Could you check a few things on this model? Use its own coordinates, in mm. Coordinates: 2 decimals unless noted, no trailing zeros. Loops run counter-clockwise (first coordinate to the right, second up) from the corner with the lowest first, then second, coordinate; pieces in that order, holes last. Notation, with made-up numbers: (21, 63) - (74, 63) arc R30 cw to (74, 97) - close; hole circle Ø1 at (75.25, 54.25). An arc over 180 degrees is marked (long way). One line per item, written item: value. Start each with the question number.
(1) If I drill on line 1 along Y through (x, z) = (1324, 0.2); line 2 along X through (y, z) = (-100.25, 1.1); line 3 along X through (y, z) = (-99.25, 0.5), over which ranges is the centre line in solid material (lowest first)? Write a range as from..to.
(2) I'm going to push flat-ended pins straight in: P1, Ø0.9, axis at x = 1324, z = 2, coming from the +Y side; P2, Ø1.5, axis at x = 1284.5, z = 2, coming from the -Y side. Where does each tip first touch, or does it pass through?
(3) If we section it at C-C on x = 1315: Write out the boundary of the cut face in (y, z), then the cut area to 3 significant figures.
(4) If we section it at A-A on z = 0.55: Write out the boundary of the cut face in (x, y).
(5) If we section it at B-B on x = 1269: Write out the boundary of the cut face in (y, z), then the cut area to 3 significant figures.
```python
from build123d import *

# Parameters (mm, degrees)
SKETCH1_R          = 2.314653827
BASE_EXTRUDE_DEPTH = 3


with BuildPart() as part:
    # Sketch1 → Base-Extrude (new body)
    with BuildSketch(Plane.XY):
        with BuildLine():
            Line((1237.912051302, -106.965442143), (1245.987496986, -95.560571197))
            ThreePointArc((1245.987496986, -95.560571197), (1253.509408231, -96.263863256), (1254.634364731, -103.73435463))
            Line((1254.634364731, -103.73435463), (1304.653724872, -103.73435463))
            Line((1304.653724872, -103.73435463), (1317.227321876, -96.706912395))
            Line((1317.227321876, -96.706912395), (1326.560817804, -96.706912395))
            Line((1326.560817804, -96.706912395), (1329.452389013, -100.73435463))
            Line((1329.452389013, -100.73435463), (1321.620543519, -100.73435463))
            Line((1321.620543519, -100.73435463), (1321.620543519, -103.73435463))
            Line((1321.620543519, -103.73435463), (1356.049186006, -103.73435463))
            ThreePointArc((1356.049186006, -103.73435463), (1359.51702166, -102.336314635), (1361.045588138, -98.92400098))
            Line((1361.045588138, -98.92400098), (1361.062528583, -98.477689842))
            Line((1361.062528583, -98.477689842), (1361.062528583, -98.158287995))
            ThreePointArc((1361.062528583, -98.158287995), (1361.210092551, -97.803620765), (1361.565683957, -97.658297951))
            Line((1361.565683957, -97.658297951), (1365.63036841, -97.683949663))
            Line((1365.63036841, -97.683949663), (1365.576237812, -106.261303213))
            Line((1365.576237812, -106.261303213), (1368.576237812, -106.280235835))
            Line((1368.576237812, -106.280235835), (1368.620142395, -99.323262365))
            Line((1368.620142395, -99.323262365), (1372.856385089, -99.349996759))
            ThreePointArc((1372.856385089, -99.349996759), (1375.348322676, -105.366702643), (1372.855935111, -111.383222141))
            Line((1372.855935111, -111.383222141), (1255.179553467, -111.383222141))
            ThreePointArc((1255.179553467, -111.383222141), (1248.674645996, -113.340903741), (1241.936111152, -114.200256171))
            Line((1241.936111152, -114.200256171), (1245.086093213, -109.745869716))
            Line((1245.086093213, -109.745869716), (1242.636669623, -108.013725357))
            Line((1242.636669623, -108.013725357), (1239.591696444, -112.41591336))
            Line((1239.591696444, -112.41591336), (1238.460322727, -110.884264434))
            Line((1238.460322727, -110.884264434), (1237.923801474, -109.055713836))
            Line((1237.923801474, -109.055713836), (1237.912051302, -106.965442143))
        make_face()
        with Locations((1249.299132798, -100.717822078)):
            Circle(SKETCH1_R, mode=Mode.SUBTRACT)
    extrude(amount=BASE_EXTRUDE_DEPTH)


solid = part.part
```
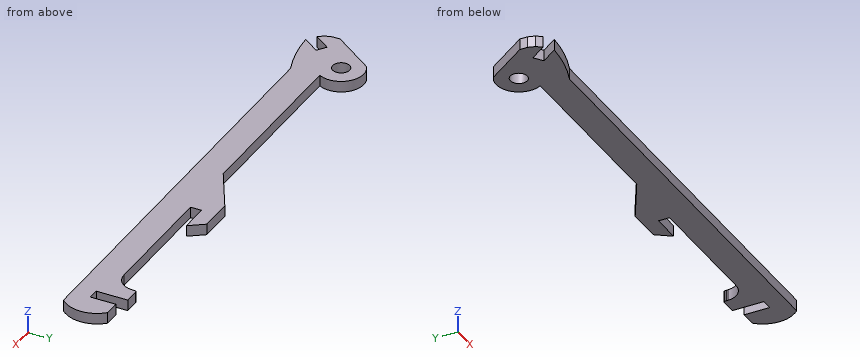
Values:
1. line 1: y = -111.38..-103.73, -100.73..-96.71
1. line 2: x = 1242.67..1247.03, 1251.57..1255.41, 1310.89..1329.1, 1360.81..1365.61, 1368.61..1373.64
1. line 3: x = 1243.38..1247.51, 1251.09..1255.25, 1312.68..1328.39, 1361.02..1365.62
2. P1: stops at y = -96.71
2. P2: stops at y = -111.38
3. outline: (-111.38, 0) - (-97.95, 0) - (-97.95, 3) - (-111.38, 3) - close
3. area: 40.3 mm2
4. outline: (1237.91, -106.97) - (1237.92, -109.06) - (1238.46, -110.88) - (1239.59, -112.42) - (1242.64, -108.01) - (1245.09, -109.75) - (1241.94, -114.2) arc R41.1 ccw to (1255.18, -111.38) - (1372.86, -111.38) arc R8.51 ccw to (1372.86, -99.35) - (1368.62, -99.32) - (1368.58, -106.28) - (1365.58, -106.26) - (1365.63, -97.68) - (1361.57, -97.66) arc R0.5 ccw to (1361.06, -98.16) - (1361.06, -98.48) - (1361.05, -98.92) arc R5 cw to (1356.05, -103.73) - (1321.62, -103.73) - (1321.62, -100.73) - (1329.45, -100.73) - (1326.56, -96.71) - (1317.23, -96.71) - (1304.65, -103.73) - (1254.63, -103.73) arc R6.13 ccw to (1245.99, -95.56) - close; hole circle Ø4.63 at (1249.3, -100.72)
5. outline: (-111.38, 0) - (-103.73, 0) - (-103.73, 3) - (-111.38, 3) - close
5. area: 22.9 mm2
